Verification items for the finished model (mm, model axes). Face numbers are marked on the shaded views. A direction names the side the tool comes from. Give positions to 0.01 mm unless a question says otherwise; leave off trailing zeros. Write each loop counter-clockwise with the first axis right and the second up, starting at its lowest first coordinate (ties: lowest second). Pieces come first, ordered by that corner, then holes.
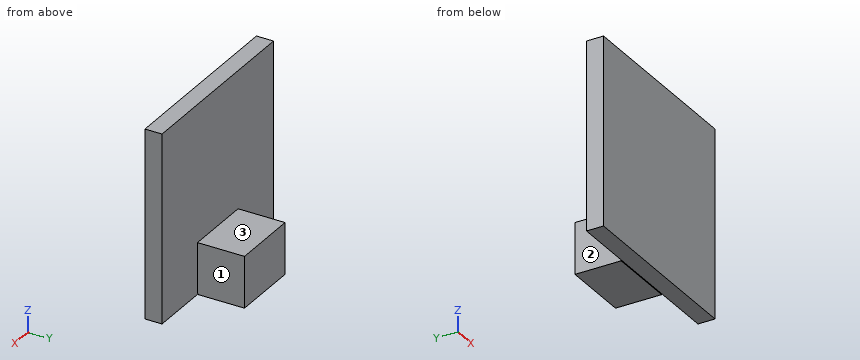
Autodesk Inventor part; units mm, degrees
ref_plane "YZ Plane" through (0, 0, 0) normal (1, 0, 0) x (0, 1, 0)
ref_plane "XZ Plane" through (0, 0, 0) normal (0, 1, 0) x (-1, 0, 0)
ref_plane "XY Plane" through (0, 0, 0) normal (0, 0, 1) x (1, 0, 0)
sketch "Sketch1" plane through (0, 0, 0) normal (0, 1, 0) x (-1, 0, 0)
  line L0 (16.6199, 13.3988) -> (-5.3801, 13.3988)
  line L1 (-5.3801, 13.3988) -> (-5.3801, -8.6012)
  line L2 (-5.3801, -8.6012) -> (16.6199, -8.6012)
  line L3 (16.6199, -8.6012) -> (16.6199, 13.3988)
  point P0 (0, 0)
  dimension "d0" = 22
  dimension "d1" = 22
extrude "Extrusion1" add sketch "Sketch1" along normal blind 2
sketch "Sketch2" plane through (0, 2, 0) normal (0, 1, 0) x (1, 0, 0)
  line L0 (5.3801, 8.6012) -> (-16.6199, 8.6012)
  line L1 (-1.6199, 8.6012) -> (-9.6199, 8.6012)
  line L2 (-9.6199, 8.6012) -> (-9.6199, 2.6012)
  line L3 (-9.6199, 2.6012) -> (-1.6199, 2.6012)
  line L4 (-1.6199, 2.6012) -> (-1.6199, 8.6012)
  line L5 (-16.6199, 8.6012) -> (-16.6199, -13.3988)
  line L6 (5.3801, -13.3988) -> (5.3801, 8.6012)
  point P0 (0, 0)
  dimension "d4" = 8
  dimension "d5" = 7
  dimension "d6" = 7
  dimension "d7" = 6
extrude "Extrusion2" add sketch "Sketch2" along normal blind 5.5
sketch "Sketch3" plane through (5.3801, 0, -8.6012) normal (0, 0, -1) x (-1, 0, 0)
  line L0 (7, 2) -> (15, 2)
  line L1 (15, 2) -> (15, 7.5)
  line L2 (7, 2) -> (15, 2)
  line L3 (15, 2) -> (15, 2.1)
  line L4 (15, 2.1) -> (7, 2.1)
  line L5 (7, 2.1) -> (7, 2)
  point P0 (5.3801, 0)
  dimension "d10" = 0.1
extrude "Extrusion3" cut sketch "Sketch3" against normal blind 0.1
properties part number "battery connector"
Item 1: Sectioned sample at B-B on z = 5. Record the cut outline in (x, y), then the cut area to 3 significant figures.
Answer key:
outline: (-16.62, 0) - (5.38, 0) - (5.38, 2) - (-16.62, 2) - close
area: 44.0 mm2
Item 2: Scan lines: line 1 along Y through (x, z) = (-9, 5); line 2 along X through (y, z) = (3.5, -6.5); line 3 along Z through (x, y) = (-8.75, 5.5). Record each from-to range of solid material in increasing order.
Answer key:
line 1: y = 0 to 2
line 2: x = -9.62 to -1.62
line 3: z = -8.6 to -2.6
Item 3: Sectioned sample at C-C on y = 5.25. Record the cut outline in (x, z).
Answer key:
outline: (-9.62, -8.6) - (-1.62, -8.6) - (-1.62, -2.6) - (-9.62, -2.6) - close
Item 4: Sectioned sample at A-A on x = -9.25. Record the cut outline in (y, z), then the cut area to 3 significant figures.
Answer key:
outline: (0, -8.6) - (2, -8.6) - (2, -8.5) - (2.1, -8.5) - (2.1, -8.6) - (7.5, -8.6) - (7.5, -2.6) - (2, -2.6) - (2, 13.4) - (0, 13.4) - close
area: 77.0 mm2
Item 5: Depth check by flat-ended pin: pin 1 (4.5 mm diameter, centred on x = -6.5, y = 3.5, fed in from +Z); pin 2 (3 mm diameter, centred on x = -5.5, y = 4, fed in from +Z); pin 3 (1.6 mm diameter, centred on y = 4.5, z = -5.5, fed in from -X); pin 4 (11 mm diameter, centred on x = -8, z = 7, fed in from +Y). Enter the tip coordinate at first touch or a pass-through.
Answer key:
pin 1: stops at z = 13.4
pin 2: stops at z = -2.6
pin 3: stops at x = -9.62
pin 4: stops at y = 2
Item 6: Set-up check for the marked faces 1, 2 and 3: record each of +Z, -Z, +X, -X, +Y, -Y from which the full face is reachable in a straight line by a thin tool's end or side.
Answer key:
face 1: +Z, -Z, +X, +Y
face 2: +Z, -Z, -X, +Y
face 3: +Z, +X, -X, +Y
